```python
from build123d import *

# Parameters (mm, degrees)
SKETCH_1_W                   = 80
SKETCH_1_H                   = 80
EXTRUDE_1_DEPTH              = 10
SKETCH_11_W                  = 10
SKETCH_11_H                  = 10
EXTRUDE_3_DEPTH              = 10
HOLE_WIZARD_M4_2_D           = 3.3
HOLE_WIZARD_M4_2_DEPTH       = 68
HOLE_WIZARD_M5_1_D           = 5.5
HOLE_WIZARD_M5_1_DEPTH       = 10
HOLE_WIZARD_M5_1_CSINK_D     = 10.4
HOLE_WIZARD_M5_1_CSINK_ANGLE = 90
HOLE_WIZARD_M6_1_D           = 5
HOLE_WIZARD_M6_1_DEPTH       = 10
HOLE_WIZARD_M6_1_CSINK_D     = 6.05
HOLE_WIZARD_M6_1_CSINK_ANGLE = 90
MIRROR_2_COPY_1_SKETCH_W     = 10
MIRROR_2_COPY_1_SKETCH_H     = 10
MIRROR_2_COPY_1_DEPTH        = 10
MIRROR_2_COPY_2_D            = 3.3
MIRROR_2_COPY_2_DEPTH        = 68
CHAMFER_1_SIZE               = 1


with BuildPart() as part:
    # 스케치1 → 보스-돌출1 (new body)
    with BuildSketch(Plane.XY):
        Rectangle(SKETCH_1_W, SKETCH_1_H)
    extrude(amount=EXTRUDE_1_DEPTH)

    # 스케치11 → 보스-돌출3 (add)
    with BuildSketch(Plane(origin=(0, 0, 0), x_dir=(-1, 0, 0), z_dir=(0, 0, -1))):
        with Locations((29, 29)):
            Rectangle(SKETCH_11_W, SKETCH_11_H)
    extrude_3 = extrude(amount=EXTRUDE_3_DEPTH)

    # M4 나사 구멍2
    with Locations(Plane(origin=(0, 34, 0), x_dir=(1, 0, 0), z_dir=(0, 1, 0))):
        with Locations((-29, 5)):
            hole_wizard_m4_2 = Hole(HOLE_WIZARD_M4_2_D / 2, depth=HOLE_WIZARD_M4_2_DEPTH)

    # M5 접시 머리 나사용 카운터싱크1
    with Locations(Plane.XY.offset(10)):
        with Locations((-6.75, 11.691342951), (-13.5, 0), (-6.75, -11.691342951), (6.75, -11.691342951), (13.5, 0), (6.75, 11.691342951)):
            CounterSinkHole(HOLE_WIZARD_M5_1_D / 2, HOLE_WIZARD_M5_1_CSINK_D / 2, depth=HOLE_WIZARD_M5_1_DEPTH, counter_sink_angle=HOLE_WIZARD_M5_1_CSINK_ANGLE)

    # M6 나사 구멍1
    with Locations(Plane.XY.offset(10)):
        with Locations((-19, -19), (19, -19), (19, 19), (-19, 19)):
            CounterSinkHole(HOLE_WIZARD_M6_1_D / 2, HOLE_WIZARD_M6_1_CSINK_D / 2, depth=HOLE_WIZARD_M6_1_DEPTH, counter_sink_angle=HOLE_WIZARD_M6_1_CSINK_ANGLE)

    # 대칭 복사1: 보스-돌출3, M4 나사 구멍2 across plane
    add(extrude_3.mirror(Plane(origin=(0, 0, 0), x_dir=(0, 0, 1), z_dir=(1, 0, 0))))
    add(hole_wizard_m4_2.mirror(Plane(origin=(0, 0, 0), x_dir=(0, 0, 1), z_dir=(1, 0, 0))), mode=Mode.SUBTRACT)

    # 대칭 복사2: 보스-돌출3, M4 나사 구멍2 across plane
    add(extrude_3.mirror(Plane.ZX))
    add(hole_wizard_m4_2.mirror(Plane.ZX), mode=Mode.SUBTRACT)

    # 대칭 복사2 copy 1 sketch → 대칭 복사2 copy 1 (add)
    with BuildSketch(Plane(origin=(0, 0, 0), x_dir=(1, 0, 0), z_dir=(0, 0, -1))):
        with Locations((29, 29)):
            Rectangle(MIRROR_2_COPY_1_SKETCH_W, MIRROR_2_COPY_1_SKETCH_H)
    extrude(amount=MIRROR_2_COPY_1_DEPTH)

    # 대칭 복사2 copy 2
    with Locations(Plane(origin=(0, -34, 0), x_dir=(-1, 0, 0), z_dir=(0, -1, 0))):
        with Locations((-29, 5)):
            Hole(MIRROR_2_COPY_2_D / 2, depth=MIRROR_2_COPY_2_DEPTH)

    # 모따기1
    chamfer_1_edges = [part.edges().sort_by_distance(p)[0] for p in [
        (34, 34, -5),
        (34, -34, -5),
        (-34, -34, -5),
        (-34, 34, -5),
    ]]
    chamfer(chamfer_1_edges, length=CHAMFER_1_SIZE)


solid = part.part
```
Source: CAD feature listing. Evaluate the final solid. Frame: model axes, mm. A direction names the side the tool comes from. Give positions to 0.01 mm unless a question says otherwise; leave off trailing zeros. Loops run counter-clockwise (first coordinate to the right, second up) from the corner with the lowest first, then second, coordinate; pieces in that order, holes last. Notation, with made-up numbers: (88.5, 78.5) -> (127.5, 78.5) arc R25 ccw to (127.5, 91.5) -> close; hole circle Ø7 at (17, 85). An arc over 180 degrees is marked (long way). Put each result on its own line as item: value. Start each with the question number.
1) Cut plane B-B (x = -29). Return loops of the section in (y, z), then the cut area to 3 significant figures.
2) Material intervals for probe 1 along Y at (x, z) = (6.75, 2.5); probe 2 along X at (y, z) = (0, 2); probe 3 along Y at (x, z) = (19, 6), sorted ascending.
3) Contact query for flat-ended pins moving along their axis: P1, Ø10, axis at x = 28, z = -6, coming from the +Y side; P2, Ø8, axis at x = -21, y = 10, coming from the -Z side; P3, Ø3.5, axis at x = 6.75, y = 11.69, coming from the -Z side; P4, Ø12, axis at x = -22, z = -5, coming from the +Y side. Output: stop coordinate, or through.
4) Draft query along X for faces 6 (the face through (-34, -28, -5)), 7 (the face through (-1, -40, 5)), 8 (the face through (5.48, 9.25, 3.72)). Return one class per face: released by +X, released by -X, zero draft, split by the parting line, or undercut.
5) Reachability of faces 1 (the face through (34, -28, -5)), 2 (the face through (-27, -34, -4)), 3 (the face through (27, 34, -4)), 4 (the face through (-24, -29, -5)), 5 (the face through (20.84, 20.69, 4.67)) from +Z, -Z, +X, -X, +Y, -Y: full face, straight path, thin tool, end or side. Return the list, or none.
6) Cut plane D-D (y = 26.5). Return loops of the section in (x, z).
7) Cut plane A-A (z = -8.5). Return loops of the section in (x, y).
8) Cut plane C-C (y = -19). Return loops of the section in (x, z) (3 decimals).
Results are:
1. outline: (-40, 0) -> (-34, 0) -> (-34, -3.35) -> (-24, -3.35) -> (-24, 0) -> (24, 0) -> (24, -3.35) -> (34, -3.35) -> (34, 0) -> (40, 0) -> (40, 10) -> (-40, 10) -> close; (-34, -10) -> (-24, -10) -> (-24, -6.65) -> (-34, -6.65) -> close; (24, -10) -> (34, -10) -> (34, -6.65) -> (24, -6.65) -> close
1. area: 934 mm2
2. probe 1: y = -40 to -14.44, -8.94 to 8.94, 14.44 to 40
2. probe 2: x = -40 to -16.25, -10.75 to 10.75, 16.25 to 40
2. probe 3: y = -40 to -21.5, -16.5 to 16.5, 21.5 to 40
3. P1: stops at y = 34
3. P2: stops at z = 0
3. P3: passes through
3. P4: stops at y = 40
4. face 6: released by -X
4. face 7: zero draft
4. face 8: undercut
5. face 1: -Z, +X, +Y, -Y
5. face 2: -Z, +X, -X, -Y
5. face 3: -Z, +X, -X, +Y
5. face 4: -Z, +Y, -Y
5. face 5: +Z, -Z
6. outline: (-40, 0) -> (-34, 0) -> (-34, -10) -> (-24, -10) -> (-24, 0) -> (24, 0) -> (24, -10) -> (34, -10) -> (34, 0) -> (40, 0) -> (40, 10) -> (-40, 10) -> close; hole circle Ø3.3 at (-29, -5); hole circle Ø3.3 at (29, -5)
7. outline: (-34, -33) -> (-33, -34) -> (-24, -34) -> (-24, -24) -> (-34, -24) -> close; (-34, 24) -> (-24, 24) -> (-24, 34) -> (-33, 34) -> (-34, 33) -> close; (24, -34) -> (33, -34) -> (34, -33) -> (34, -24) -> (24, -24) -> close; (24, 24) -> (34, 24) -> (34, 33) -> (33, 34) -> (24, 34) -> close
8. outline: (-40, 0) -> (-21.5, 0) -> (-21.5, 9.475) -> (-22.025, 10) -> (-40, 10) -> close; (-16.5, 0) -> (16.5, 0) -> (16.5, 9.475) -> (15.975, 10) -> (-15.975, 10) -> (-16.5, 9.475) -> close; (21.5, 0) -> (40, 0) -> (40, 10) -> (22.025, 10) -> (21.5, 9.475) -> close
